Input: dimensioned drawing with shaded views. Units: mm. Origin: part minimum x, y, z. Coordinates: 2 decimals unless noted, no trailing zeros. Order: outer loops, then holes, each group sorted by start corner. A loop starts at its lowest first (then second) coordinate and runs counter-clockwise, first axis right, second up. Notation, with made-up numbers: (24.5, 41) -> (43.5, 41) arc R9 ccw to (43.5, 49) -> close; hole circle Ø10 at (80.5, 9). An arc over 180 degrees is marked (long way). Put each result on its own line as item: value.
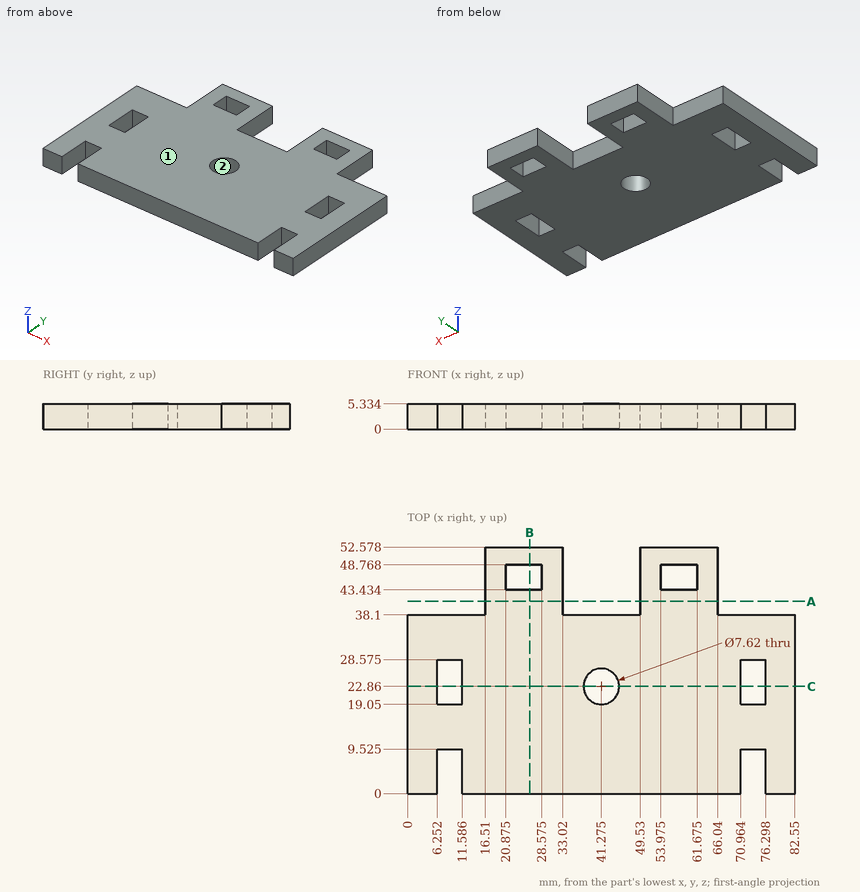
1. First-contact query: pin 1 (2.5 mm diameter, centred on x = 73.5, z = 2, fed in from +Y); pin 2 (2.5 mm diameter, centred on y = 45.5, z = 3, fed in from -X); pin 3 (2.5 mm diameter, centred on y = 43, z = 4, fed in from +X). Flat tips, straight axial feed; report the tip coordinate or a pass-through.
Numbers:
pin 1: stops at y = 38.1
pin 2: stops at x = 16.51
pin 3: stops at x = 66.04
2. Ray query, line 1 along X through (y, z) = (47, 2.3) (1 decimal); line 2 along X through (y, z) = (39, 1.3); line 3 along Y through (x, z) = (23, 1.45). Return the intervals inside material, ascending.
Numbers:
line 1: x = 16.5 to 20.9, 28.6 to 33, 49.5 to 54, 61.7 to 66
line 2: x = 16.51 to 33.02, 49.53 to 66.04
line 3: y = 0 to 43.43, 48.77 to 52.58
3. Pull-direction query (X, two-part tool) for the marked faces 1 and 2; classes: pulls with the +X half, pulls with the -X half, needs draft (parallel to the pull), parting line crosses it, or undercut.
Numbers:
face 1: needs draft
face 2: undercut
4. Cut plane C-C on y = 22.86. Count the separate pieces of the cut face and the enclosed holes in it, plus the area to 3 significant figures.
Numbers:
separate pieces: 4
enclosed holes: 0
area: 343 mm2
5. Cut plane A-A on y = 41. Output: boundary loops of the cut face in (x, z).
Numbers:
outline: (16.51, 0) -> (33.02, 0) -> (33.02, 5.33) -> (16.51, 5.33) -> close; (49.53, 0) -> (66.04, 0) -> (66.04, 5.33) -> (49.53, 5.33) -> close
6. Cut plane B-B on x = 26. Output: boundary loops of the cut face in (y, z), plus the area to 3 significant figures.
Numbers:
outline: (0, 0) -> (43.43, 0) -> (43.43, 5.33) -> (0, 5.33) -> close; (48.77, 0) -> (52.58, 0) -> (52.58, 5.33) -> (48.77, 5.33) -> close
area: 252 mm2
